```python
from build123d import *

# Parameters (mm, degrees)
F_4_CLEARANCE_HOLE1_D = 2.9464


with BuildPart() as part:
    # Sketch2 → Revolve1 (revolve)
    with BuildSketch(Plane(origin=(0, 0, 0), x_dir=(0, 0, -1), z_dir=(1, 0, 0)), mode=Mode.PRIVATE) as revolve1_sk:
        Polygon((0, 0), (15.875, 0), (15.875, 17.280736743), (15.875, 19.9898), (12.7, 19.9898), (12.7, 13.931139367), (7.62, 10.9982), (7.62, 8.9662), (0, 8.9662), align=None)
    revolve(revolve1_sk.sketch.rotate(Axis((0, 0, 0), (0, 0, -1)), 90), axis=Axis((0, 0, 0), (0, 0, -1)))

    # #4 Clearance Hole1 (through all)
    with Locations(Plane(origin=(0, 0, -15.875), x_dir=(-1, 0, 0), z_dir=(0, 0, -1))):
        with Locations((0, 16.8275), (-16.8275, 0), (16.8275, 0), (0, -16.8275)):
            Hole(F_4_CLEARANCE_HOLE1_D / 2)


solid = part.part
```
Read the model definition and answer for the solid it produces. Units are mm, in the model's axes. A direction names the side the tool comes from. Give positions to 0.01 mm unless a question says otherwise; leave off trailing zeros. Order: outer loops, then holes, each group sorted by start corner. A loop starts at its lowest first (then second) coordinate and runs counter-clockwise, first axis right, second up.
(1) Find section C-C (z = -2.25). Give the vertices of the cut face in (x, y), plus the area to 3 significant figures.
(2) For faces 1 (the flat face through (2, 9, -7.62)), 2 (the flat face through (0, 0, 0)), determine the directions among +Z, -Z, +X, -X, +Y, -Y from which every point of the face is accessible in a straight line to the end or side of a thin tool.
(3) Find section D-D (z = -13.5). Give the vertices of the cut face in (x, y), plus the area to 3 significant figures.
(4) Given pin 1 (3 mm diameter, centred on x = -6, y = -13, fed in from +Z); pin 2 (3 mm diameter, centred on x = 2.5, z = -3, fed in from +Y); pin 3 (6 mm diameter, centred on x = 13.5, z = -9, fed in from -Y); pin 4 (2.5 mm diameter, centred on x = 16.83, y = 0, fed in from -Z), each flat-ended and moving along its own axis, determine where each tip first touches the part or whether it passes through.
(5) Find section A-A (y = 0). Give the vertices of the cut face in (x, z) (3 decimals), plus the area to 3 significant figures.
(6) Straight lines are drawn through the part: L1, parallel to Y at x = 0, z = -14.55; L2, parallel to Z at x = 5, y = 14 (3 decimals); L3, parallel to Z at x = -9, y = 1 (3 decimals). For each, find the intervals that lie inside material, in ascending order.
(7) For a pull along Y with two mould halves and no side action, classify faces 3 (the flat face through (-13.42, 4.35, -12.7)), 4 (the cylindrical face through (-0.192, -15.367, -14.265)), 5 (the cylindrical face through (-15.863, 12.163, -14.265)) as released by +Y, released by -Y, zero draft, split by the parting line, or undercut.
Result sheet:
1. outline: circle Ø17.93 at (0, 0)
1. area: 253 mm2
2. face 1: +Z
2. face 2: +Z, +X, -X, +Y, -Y
3. outline: circle Ø39.98 at (0, 0); hole circle Ø2.95 at (-16.83, 0); hole circle Ø2.95 at (0, -16.83); hole circle Ø2.95 at (0, 16.83); hole circle Ø2.95 at (16.83, 0)
3. area: 1,230 mm2
4. pin 1: stops at z = -10.77
4. pin 2: stops at y = 8.91
4. pin 3: stops at y = -6.45
4. pin 4: passes through
5. outline: (-19.99, -15.875) - (-18.301, -15.875) - (-18.301, -12.7) - (-19.99, -12.7) - close; (-15.354, -15.875) - (15.354, -15.875) - (15.354, -12.7) - (13.931, -12.7) - (10.998, -7.62) - (8.966, -7.62) - (8.966, 0) - (-8.966, 0) - (-8.966, -7.62) - (-10.998, -7.62) - (-13.931, -12.7) - (-15.354, -12.7) - close; (18.301, -15.875) - (19.99, -15.875) - (19.99, -12.7) - (18.301, -12.7) - close
5. area: 372 mm2
6. L1: y = -19.99 to -18.3, -15.35 to 15.35, 18.3 to 19.99
6. L2: z = -15.875 to -12.7
6. L3: z = -15.875 to -7.62
7. face 3: zero draft
7. face 4: undercut
7. face 5: split by the parting line
